Part print with two shaded views. Sizes in mm from the minimum x, y, z corner. A direction names the side the tool comes from. Round coordinates to 2 decimals unless told otherwise and drop trailing zeros. Write each loop counter-clockwise with the first axis right and the second up, starting at its lowest first coordinate (ties: lowest second). Pieces come first, ordered by that corner, then holes.
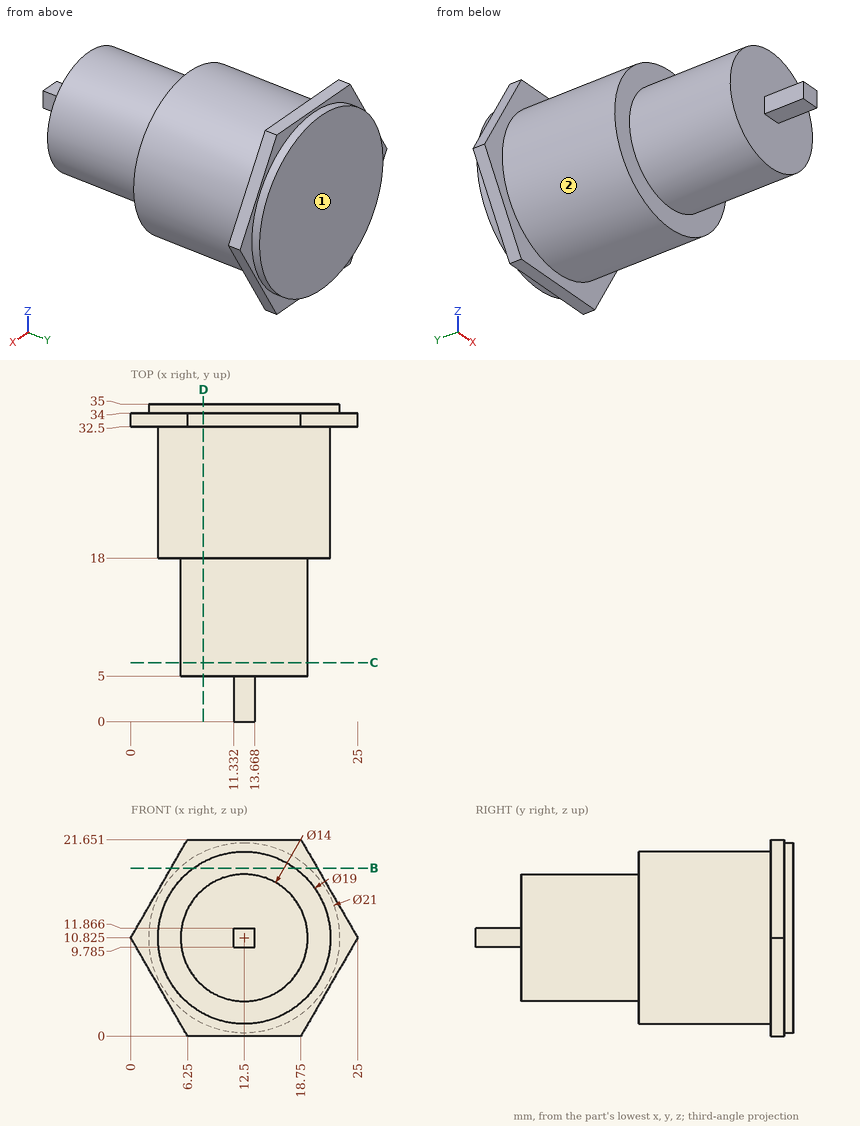
Q1. Cut at B-B on z = 18.5. Write the cut outline in (x, y), plus the area to 3 significant figures.
Values follow:
outline: (4.43, 32.5) - (6.9, 32.5) - (6.9, 18) - (18.1, 18) - (18.1, 32.5) - (20.57, 32.5) - (20.57, 34) - (19.67, 34) - (19.67, 35) - (5.33, 35) - (5.33, 34) - (4.43, 34) - close
area: 201 mm2
Q2. Wall check: L1, parallel to Y at x = 13.75, z = 4.5; L2, parallel to Y at x = 4, z = 6; L3, parallel to X at y = 14.5, z = 11. Give the ranges that are in metal, low to high.
Values follow:
L1: y = 5 to 35
L2: y = 32.5 to 35
L3: x = 5.5 to 19.5
Q3. Drop flat-ended pins along their axis: pin 1 (1.9 mm diameter, centred on x = 12, y = 3.5, fed in from -Z) (1 decimal); pin 2 (6 mm diameter, centred on x = 21, y = 26.5, fed in from +Z); pin 3 (4 mm diameter, centred on x = 9, z = 7.5, fed in from -Y). Give the stop position or say it passes through.
Values follow:
pin 1: stops at z = 9.8
pin 2: stops at z = 18.57
pin 3: stops at y = 5
Q4. Cut at D-D on x = 8. Write the cut outline in (y, z).
Values follow:
outline: (5, 5.46) - (18, 5.46) - (18, 2.46) - (32.5, 2.46) - (32.5, 0) - (34, 0) - (34, 1.34) - (35, 1.34) - (35, 20.31) - (34, 20.31) - (34, 21.65) - (32.5, 21.65) - (32.5, 19.19) - (18, 19.19) - (18, 16.19) - (5, 16.19) - close
Q5. Which spindle directions (+Z, -Z, +X, -X, +Y, -Y) get a long thin tool onto all of the face, cutting with end or side? Do the marked faces 1 and 2. Say none if no direction does.
Values follow:
face 1: +Z, -Z, +X, -X, +Y
face 2: -Y
Q6. Cut at C-C on y = 6.5. Write the cut outline in (x, z) (1 decimal), plus the area to 3 significant figures.
Values follow:
outline: circle Ø14 at (12.5, 10.8)
area: 154 mm2
